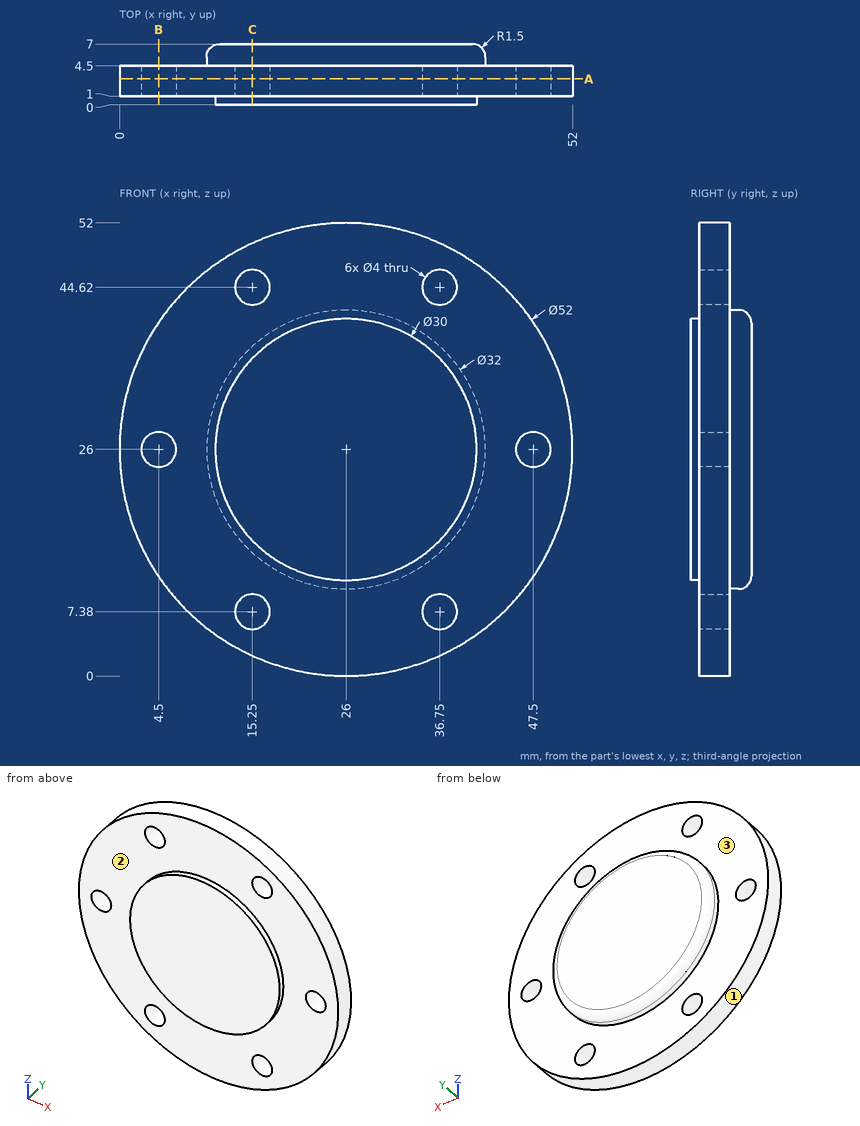
Geometry check sheet. Reference: drawing and pictorial views, mm from the part's lowest x, y, z. A direction names the side the tool comes from. Coordinates: 2 decimals unless noted, no trailing zeros. Order: outer loops, then holes, each group sorted by start corner. A loop starts at its lowest first (then second) coordinate and runs counter-clockwise, first axis right, second up. Notation, with made-up numbers: (-7, -15.5) - (36, -15.5) arc R31 cw to (36, 15.5) - close; hole circle Ø8 at (49.25, 87). An arc over 180 degrees is marked (long way). One line per item, written item: value.
(1) Sectioned sample at A-A (y = 3). Enter the section's corners in (x, z), and give its area (3 significant figures).
Data:
outline: circle Ø52 at (26, 26); hole circle Ø4 at (4.5, 26); hole circle Ø4 at (15.25, 7.38); hole circle Ø4 at (15.25, 44.62); hole circle Ø4 at (36.75, 7.38); hole circle Ø4 at (36.75, 44.62); hole circle Ø4 at (47.5, 26)
area: 2,050 mm^2
(2) Thickness scan on probe 1 along X at (y, z) = (3.55, 26); probe 2 along X at (y, z) = (4, 9) (1 decimal); probe 3 along Z at (x, y) = (36.75, 1.85) (1 decimal). Record the ranges inside material, lowest first. Write a range as from..to.
Data:
probe 1: x = 0..2.5, 6.5..45.5, 49.5..52
probe 2: x = 6.3..14.1, 16.4..35.6, 37.9..45.7
probe 3: z = 2.3..5.4, 9.4..42.6, 46.6..49.7
(3) Access from +Z, -Z, +X, -X, +Y, -Y to the whole of each face (thin tool, end or side, straight path). Record for the marked faces 1, 2 and 3.
Data:
face 1: +Y, -Y
face 2: -Y
face 3: +Y
(4) Depth check by flat-ended pin: pin 1 Ø6.5 at (x, z) = (36.75, 44.62) entering from +Y; pin 2 Ø4 at (x, y) = (32.5, 2.5) entering from +Z; pin 3 Ø4 at (x, y) = (45, 2.5) entering from -Z; pin 4 Ø3.5 at (x, z) = (15.25, 7.38) entering from -Y. Enter the tip coordinate at first touch or a pass-through.
Data:
pin 1: stops at y = 4.5
pin 2: stops at z = 51.61
pin 3: stops at z = 6.33
pin 4: passes through
(5) Sectioned sample at B-B (x = 4.5). Enter the section's corners in (y, z).
Data:
outline: (1, 11.38) - (4.5, 11.38) - (4.5, 24) - (1, 24) - close; (1, 28) - (4.5, 28) - (4.5, 40.62) - (1, 40.62) - close
(6) Sectioned sample at C-C (x = 15.25). Count the separate pieces of the cut face and the enclosed holes in it.
Data:
separate pieces: 3
enclosed holes: 0
